```python
from build123d import *

# Parameters (mm, degrees)
ESQUISSE1_R             = 1.05
ESQUISSE1_R_2           = 2.25
BOSS_EXTRU_1_DEPTH      = 5
ENL_V_MAT_EXTRU_1_DEPTH = 2.2
CONG_1_R                = 10


with BuildPart() as part:
    # Esquisse1 → Boss.-Extru.1 (new body)
    with BuildSketch(Plane(origin=(0, 0, 0), x_dir=(1, 0, 0), z_dir=(0, 1, 0))):
        with BuildLine():
            Line((-6.34428877, 4), (-55, 4))
            ThreePointArc((-55, 4), (-59, 0), (-55, -4))
            Line((-55, -4), (-6.34428877, -4))
            ThreePointArc((-6.34428877, -4), (0, -7.5), (6.34428877, -4))
            Line((6.34428877, -4), (55, -4))
            ThreePointArc((55, -4), (59, 0), (55, 4))
            Line((55, 4), (6.34428877, 4))
            ThreePointArc((6.34428877, 4), (0, 7.5), (-6.34428877, 4))
        make_face()
        with Locations(Location((-3, 4.5, 0), (0, 0, 270))):
            Circle(ESQUISSE1_R, mode=Mode.SUBTRACT)
        with Locations(Location((3, -4.5, 0), (0, 0, 270))):
            Circle(ESQUISSE1_R, mode=Mode.SUBTRACT)
        with Locations(Location((0, 0, 0), (0, 0, 270))):
            Circle(ESQUISSE1_R_2, mode=Mode.SUBTRACT)
        with BuildLine():
            Line((-22.5, -1.5), (-52.5, -1.5))
            ThreePointArc((-52.5, -1.5), (-54, 0), (-52.5, 1.5))
            Line((-52.5, 1.5), (-22.5, 1.5))
            ThreePointArc((-22.5, 1.5), (-21, 0), (-22.5, -1.5))
        make_face(mode=Mode.SUBTRACT)
        with BuildLine():
            Line((22.5, -1.5), (52.5, -1.5))
            ThreePointArc((52.5, -1.5), (54, 0), (52.5, 1.5))
            Line((52.5, 1.5), (22.5, 1.5))
            ThreePointArc((22.5, 1.5), (21, 0), (22.5, -1.5))
        make_face(mode=Mode.SUBTRACT)
    extrude(amount=BOSS_EXTRU_1_DEPTH)

    # Esquisse2 → Enlèv. mat.-Extru.1 (cut)
    with BuildSketch(Plane(origin=(0, 5, 0), x_dir=(1, 0, 0), z_dir=(0, 1, 0))):
        with BuildLine():
            Line((-14, 2.15), (-2.323252031, 2.75))
            ThreePointArc((-2.323252031, 2.75), (0, 3.6), (2.323252031, 2.75))
            Line((2.323252031, 2.75), (14, 2.15))
            ThreePointArc((14, 2.15), (16.15, 0), (14, -2.15))
            Line((14, -2.15), (2.323252031, -2.75))
            ThreePointArc((2.323252031, -2.75), (0, -3.6), (-2.323252031, -2.75))
            Line((-2.323252031, -2.75), (-14, -2.15))
            ThreePointArc((-14, -2.15), (-16.15, 0), (-14, 2.15))
        make_face()
    extrude(amount=-ENL_V_MAT_EXTRU_1_DEPTH, mode=Mode.SUBTRACT)

    # Congé1
    cong_1_edges = [part.edges().sort_by_distance(p)[0] for p in [
        (6.34428877, 2.5, 4),
        (-6.34428877, 2.5, 4),
        (-6.34428877, 2.5, -4),
        (6.34428877, 2.5, -4),
    ]]
    fillet(cong_1_edges, radius=CONG_1_R)


solid = part.part
```
Can you work these out from the model? Positions are in its coordinate system, mm. A direction names the side the tool comes from. Coordinates: 2 decimals unless noted, no trailing zeros. Loops run counter-clockwise (first coordinate to the right, second up) from the corner with the lowest first, then second, coordinate; pieces in that order, holes last. Notation, with made-up numbers: (59.25, 9.5) -> (101.25, 9.5) arc R26 cw to (101.25, 34.5) -> close; hole circle Ø11 at (0.5, 15.5). An arc over 180 degrees is marked (long way). Put each result on its own line as item: value. Start each with the question number.
Q1. I want a section at B-B (y = 3.6). Count the separate pieces of the cut face and the enclosed holes in it, plus the area to 3 significant figures.
Q2. Thinking about a two-plate mould opening in X: for faces 6 (the face through (7.295, 2.535, 4.528)), 7 (the face through (8.08, 3.915, -2.454)), 8 (the face through (0.676, 1.38, 2.146)), 9 (the face through (-33, 2, 4)), which applies, pulls with the +X half, pulls with the -X half, needs draft (parallel to the pull), parting line crosses it, or undercut?
Q3. I'm going to push flat-ended pins straight in: P1, Ø2.5, axis at x = -39.5, y = 3.5, coming from the -Z side; P2, Ø1, axis at y = 2, z = -2.5, coming from the +X side; P3, Ø5, axis at x = 0, z = 0, coming from the +Y side. Where does each tip first touch, or does it pass through?
Q4. I want a section at C-C (x = -30). Write out the boundary of the cut face in (y, z), plus the area to 3 significant figures.
Q5. For faces 1 (the face through (7.295, 2.535, -4.528)), 2 (the face through (37, 2, 1.5)), 3 (the face through (-32, 2, -4)), 4 (the face through (32, 2, 4)), 5 (the face through (16.15, 3.92, -0.05)), which set-ups out of +Z, -Z, +X, -X, +Y, -Y let a thin tool reach every point of the face, with its end or its side?
Q6. If I drill on line 1 (X direction, y = 0.9, z = 0); line 2 (X direction, y = 3.8, z = -0.25); line 3 (Z direction, x = 52, y = 2.85), over which ranges is the centre line in solid material (lowest first)? Write a range as [from, to].
Q7. I want a section at A-A (x = 0). Write out the boundary of the cut face in (y, z), plus the area to 3 significant figures.
Taken from the geometry:
1. separate pieces: 1
1. enclosed holes: 5
1. area: 639 mm2
2. face 6: pulls with the +X half
2. face 7: undercut
2. face 8: undercut
2. face 9: needs draft
3. P1: stops at z = -4
3. P2: stops at x = 58.46
3. P3: stops at y = 2.8
4. outline: (0, -4) -> (5, -4) -> (5, -1.5) -> (0, -1.5) -> close; (0, 1.5) -> (5, 1.5) -> (5, 4) -> (0, 4) -> close
4. area: 25.0 mm2
5. face 1: -Z, +X, +Y, -Y
5. face 2: +Y, -Y
5. face 3: -Z, -X, +Y, -Y
5. face 4: +Z, +X, +Y, -Y
5. face 5: +Y
6. line 1: x = [-59, -54], [-21, -2.25], [2.25, 21], [54, 59]
6. line 2: x = [-58.99, -53.98], [-21.02, -16.14], [16.14, 21.02], [53.98, 58.99]
6. line 3: z = [-4, -1.5], [1.5, 4]
7. outline: (0, -7.5) -> (5, -7.5) -> (5, -3.6) -> (2.8, -3.6) -> (2.8, -2.25) -> (0, -2.25) -> close; (0, 2.25) -> (2.8, 2.25) -> (2.8, 3.6) -> (5, 3.6) -> (5, 7.5) -> (0, 7.5) -> close
7. area: 46.6 mm2
